Design review of the part built by this model. Coordinates are the model's own, in mm. Coordinates: 2 decimals unless noted, no trailing zeros. Write each loop counter-clockwise with the first axis right and the second up, starting at its lowest first coordinate (ties: lowest second). Pieces come first, ordered by that corner, then holes. Notation, with made-up numbers: M -7.75,86.25 L 10.25,86.25 A31 cw 10.25,121.25 Z; hole C 61.25,-12.5 d8. An arc over 180 degrees is marked long. Write each question's results on one line, items separated by ' | '. Start each with the question number.
Autodesk Inventor part; units mm, degrees
ref_plane "YZ Plane" through (0, 0, 0) normal (1, 0, 0) x (0, 1, 0)
ref_plane "XZ Plane" through (0, 0, 0) normal (0, 1, 0) x (-1, 0, 0)
ref_plane "XY Plane" through (0, 0, 0) normal (0, 0, 1) x (1, 0, 0)
ref_plane "Work Plane1" through (-878.5434, 221.5358, -1189.8607) normal (0, 0, 1) x (1, 0, 0)
sketch "Sketch2" plane through (-878.5434, 221.5358, -1189.8607) normal (0, 0, 1) x (1, 0, 0)
  line L0 (431.8, -127) -> (431.8, -304.8)
  line L1 (431.8, -304.8) -> (431.8, -393.7)
  line L2 (431.8, -393.7) -> (431.8, -635)
  line L3 (431.8, -635) -> (-127, -635)
  line L4 (-127, -635) -> (-127, -304.8)
  line L5 (-127, -304.8) -> (-127, -127)
  line L6 (304.8, 0) -> (0, 0)
  arc A0 (0, 12.7) -> (-139.7, -127) centre (0, -127) ccw construction
  line L7 (0, 12.7) -> (0, 11.049)
  arc A1 (0, 11.049) -> (-138.049, -127) centre (0, -127) ccw construction
  line L8 (-138.049, -127) -> (-139.7, -127)
  arc A2 (0, -12.7) -> (-114.3, -127) centre (0, -127) ccw construction
  line L9 (-114.3, -127) -> (-115.951, -127)
  arc A3 (0, -11.049) -> (-115.951, -127) centre (0, -127) ccw construction
  line L10 (0, -11.049) -> (0, -12.7)
  arc A4 (444.5, -127) -> (304.8, 12.7) centre (304.8, -127) ccw construction
  line L11 (444.5, -127) -> (442.849, -127)
  arc A5 (442.849, -127) -> (304.8, 11.049) centre (304.8, -127) ccw construction
  line L12 (304.8, 11.049) -> (304.8, 12.7)
  arc A6 (419.1, -127) -> (304.8, -12.7) centre (304.8, -127) ccw construction
  line L13 (304.8, -12.7) -> (304.8, -11.049)
  arc A7 (420.751, -127) -> (304.8, -11.049) centre (304.8, -127) ccw construction
  line L14 (420.751, -127) -> (419.1, -127)
  line L15 (0, -127) -> (179.6051, -127) construction
  line L16 (0, -127) -> (-80.8223, -46.1777) construction
  line L17 (-81.9897, -45.0103) -> (-97.6154, -29.3846)
  line L18 (-98.7828, -28.2172) -> (-127, 0)
  arc A8 (0, 0) -> (-127, -127) centre (0, -127) ccw
  line L19 (152.4, 0) -> (152.4, -147.1377) construction
  arc A9 (431.8, -127) -> (304.8, 0) centre (304.8, -127) ccw
  line L20 (-152.4, -127) -> (-152.4, -304.8)
  line L21 (-152.4, -304.8) -> (-152.4, -635)
  line L22 (457.2, -635) -> (457.2, -393.7)
  line L23 (457.2, -393.7) -> (457.2, -304.8)
  line L24 (457.2, -304.8) -> (457.2, -127)
  arc A10 (457.2, -127) -> (304.8, 25.4) centre (304.8, -127) ccw
  line L25 (304.8, 25.4) -> (0, 25.4)
  arc A11 (0, 25.4) -> (-152.4, -127) centre (0, -127) ccw
  line L26 (-153.9875, -304.8) -> (-153.9875, -127)
  arc A12 (0, 26.9875) -> (-153.9875, -127) centre (0, -127) ccw
  line L27 (0, 26.9875) -> (304.8, 26.9875)
  arc A13 (458.7875, -127) -> (304.8, 26.9875) centre (304.8, -127) ccw
  line L28 (458.7875, -127) -> (458.7875, -304.8)
  line L29 (458.7875, -304.8) -> (458.7875, -393.7)
  line L30 (458.7875, -393.7) -> (458.7875, -635)
  line L31 (-153.9875, -635) -> (-153.9875, -304.8)
  line L32 (431.8, -635) -> (458.7875, -635)
  line L33 (-127, -635) -> (-153.9875, -635)
  point P0 (878.5434, -221.5358)
  point P1 (-89.8026, -37.1974)
  point P2 (-107.7631, -19.2369)
  point P3 (-108.8856, -18.1144)
  dimension "d1" = 25.4
  dimension "d2" = 1.5875
extrude "Extrusion2" add sketch "Sketch2" along normal blind 25.4 contours L22 L23 L24 A10 L25 A11 L18 A12 L27 A13 L28 L29 L30 L32 | L33 L31 L26 A12 L18 A11 L20 L21
properties part number "end body"
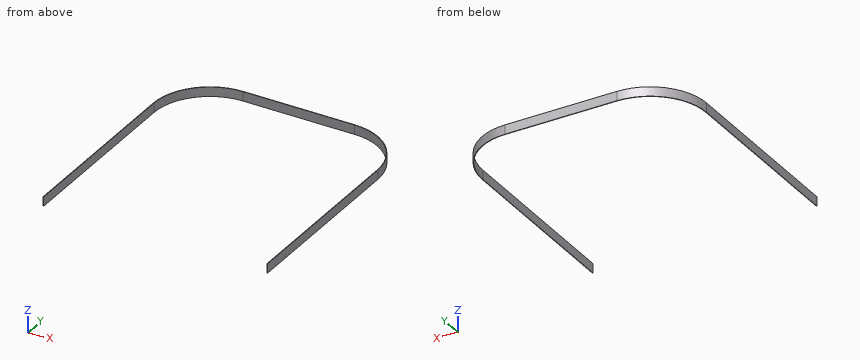
Item 1: Wall thickness on L1, parallel to X at y = -342.5, z = -1176.75; L2, parallel to Y at x = -598.5, z = -1166.5; L3, parallel to X at y = 195, z = -1170.5: over which ranges is each line inside the solid? List them lowest first.
Item 2: We need section A-A on y = -230. State the section outline as (x, z) points.
Item 3: We need section C-C on y = 154.5. State the section outline as (x, z) points, then the cut area to 3 significant figures.
Item 4: We need section B-B on z = -1174.25. State the section outline as (x, y) points (1 decimal).
Item 5: Insertion check: pin 1 Ø1 at (x, z) = (-644, -1181.5) entering from -Y; pin 2 Ø12 at (x, z) = (-557.5, -1185) entering from -Y; pin 3 Ø12 at (x, z) = (-907.5, -1177) entering from -Y. Each pin has a flat end and moves straight along its axis. Give the tip position at first contact, or say it passes through.
Item 6: We need section D-D on x = -600. State the section outline as (y, z) points.
Answer:
1) L1: x = -1032.53 to -1030.94, -421.34 to -419.76 | L2: y = 246.94 to 248.52 | L3: x = -995.24 to -993.14, -459.15 to -457.04
2) outline: M -1032.53,-1189.86 L -1030.94,-1189.86 L -1030.94,-1164.46 L -1032.53,-1164.46 Z; M -421.34,-1189.86 L -419.76,-1189.86 L -419.76,-1164.46 L -421.34,-1164.46 Z
3) outline: M -1020.38,-1189.86 L -1018.65,-1189.86 L -1018.65,-1164.46 L -1020.38,-1164.46 Z; M -433.64,-1189.86 L -431.91,-1189.86 L -431.91,-1164.46 L -433.64,-1164.46 Z | area: 87.6 mm^2
4) outline: M -1032.5,-413.5 L -1030.9,-413.5 L -1030.9,94.5 A152.4 cw -878.5,246.9 L -573.7,246.9 A152.4 cw -421.3,94.5 L -421.3,-413.5 L -419.8,-413.5 L -419.8,94.5 A154 ccw -573.7,248.5 L -878.5,248.5 A154 ccw -1032.5,94.5 Z
5) pin 1: stops at y = 246.94 | pin 2: stops at y = 245.3 | pin 3: stops at y = 242.87
6) outline: M 246.94,-1189.86 L 248.52,-1189.86 L 248.52,-1164.46 L 246.94,-1164.46 Z
